Print and shaded views of the part. All mm, measured from the part's lowest x, y and z. A direction names the side the tool comes from. Coordinates: 2 decimals unless noted, no trailing zeros. Loops run counter-clockwise (first coordinate to the right, second up) from the corner with the lowest first, then second, coordinate; pieces in that order, holes last. Notation, with made-up numbers: (-26, 54) -> (25, 54) arc R14 ccw to (25, 72) -> close; hole circle Ø5 at (-24, 3.5). An arc over 180 degrees is marked (long way). One line per question, with ' | ' between items. Start each with the question number.
1) Probe L1, parallel to X at y = 38.1, z = 23; L2, parallel to Y at x = 139.7, z = 11.5; L3, parallel to Y at x = 139, z = 25. List the from-to ranges inside material, lowest first. Write a range as from..to.
2) Cut at A-A (y = 38.1). List the corners of the cut face in (x, z) (3 decimals).
3) 3-axis set-ups, long thin cutter, end or side, ignore diameter. For the marked faces 4 and 5: which of +Z, -Z, +X, -X, +Y, -Y reach the whole face in a straight line?
4) Cut at B-B (x = 139.7). List the corners of the cut face in (y, z) (3 decimals).
5) Cut at D-D (x = 26). List the corners of the cut face in (y, z).
6) Drop flat-ended pins along their axis: pin 1 (24 mm diameter, centred on y = 23.5, z = 48, fed in from +X); pin 2 (23 mm diameter, centred on x = 41.275, z = 76.2, fed in from -Y); pin 3 (3 mm diameter, centred on y = 56, z = 64.5, fed in from +X); pin 4 (3 mm diameter, centred on x = 103, y = 25.5, fed in from +Z) (3 decimals). Give the stop position or say it passes through.
7) Cut at C-C (y = 21). List the corners of the cut face in (x, z) (3 decimals).
8) Two-plate mould, pull along Z, no slides. Class the marked faces 1, 2 and 3: released by +Z, released by -Z, zero draft, split by the parting line, or undercut.
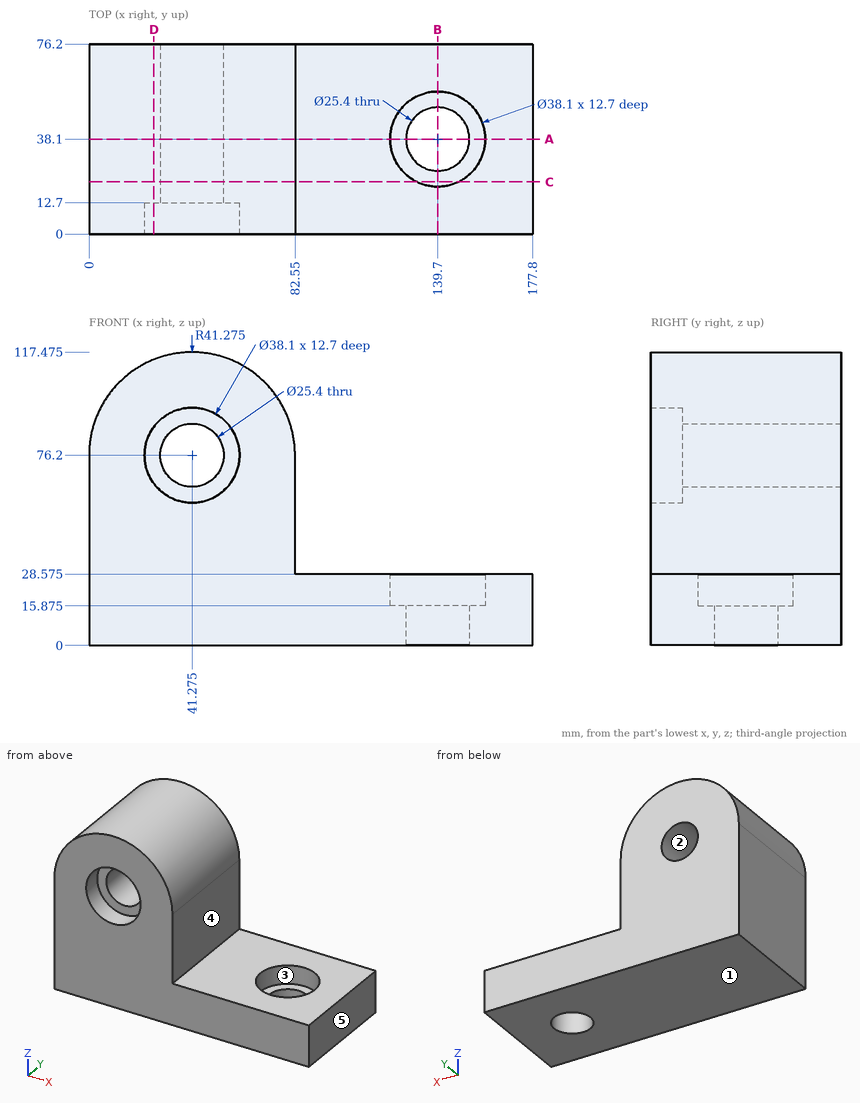
Reported:
1) L1: x = 0..120.65, 158.75..177.8 | L2: y = 0..25.4, 50.8..76.2 | L3: y = 0..19.06, 57.14..76.2
2) outline: (0, 0) -> (127, 0) -> (127, 15.875) -> (120.65, 15.875) -> (120.65, 28.575) -> (82.55, 28.575) -> (82.55, 76.2) arc R41.275 ccw to (0, 76.2) -> close; (152.4, 0) -> (177.8, 0) -> (177.8, 28.575) -> (158.75, 28.575) -> (158.75, 15.875) -> (152.4, 15.875) -> close; hole circle Ø25.4 at (41.275, 76.2)
3) face 4: +Z, +X, +Y, -Y | face 5: +Z, -Z, +X, +Y, -Y
4) outline: (0, 0) -> (25.4, 0) -> (25.4, 15.875) -> (19.05, 15.875) -> (19.05, 28.575) -> (0, 28.575) -> close; (50.8, 0) -> (76.2, 0) -> (76.2, 28.575) -> (57.15, 28.575) -> (57.15, 15.875) -> (50.8, 15.875) -> close
5) outline: (0, 0) -> (76.2, 0) -> (76.2, 114.54) -> (0, 114.54) -> (0, 87.58) -> (12.7, 87.58) -> (12.7, 64.82) -> (0, 64.82) -> close
6) pin 1: stops at x = 82.55 | pin 2: passes through | pin 3: stops at x = 82.55 | pin 4: stops at z = 28.575
7) outline: (0, 0) -> (177.8, 0) -> (177.8, 28.575) -> (148.096, 28.575) -> (148.096, 15.875) -> (131.304, 15.875) -> (131.304, 28.575) -> (82.55, 28.575) -> (82.55, 76.2) arc R41.275 ccw to (0, 76.2) -> close; hole circle Ø25.4 at (41.275, 76.2)
8) face 1: released by -Z | face 2: undercut | face 3: zero draft
